Can you work these out from the model? Positions are in its coordinate system, mm. A direction names the side the tool comes from. Coordinates: 2 decimals unless noted, no trailing zeros. Order: outer loops, then holes, each group sorted by start corner. A loop starts at its lowest first (then second) coordinate and runs counter-clockwise, first axis right, second up. Notation, with made-up numbers: (45.25, -4) -> (62.25, -4) arc R28 cw to (62.25, 21) -> close; hole circle Ø5 at (89.25, 16.5). An arc over 180 degrees is marked (long way). Answer as a JSON object with one key per item and string values. Group by question number.
(1) For pin 1 (1.9 mm diameter, centred on y = -3.5, z = 120, fed in from -X), with a flat end and sliding along its axis, tell me the tip position at first contact or that it passes through.
(2) I want a section at B-B, the plane z = 112.5. List the corners of the cut face in (x, y) for me.
(3) I want a section at C-C, the plane x = 69.5. List the corners of the cut face in (y, z) for me, plus the area to 3 significant figures.
(4) Which directions (+Z, -Z, +X, -X, +Y, -Y) give clear straight access to the entire face, cutting with the end or side of a thin tool? Please do faces 1 (the flat face through (44, -6.35, 155)), 2 (the flat face through (6.35, -3, 91)).
(5) I want a section at A-A, the plane y = -4. List the corners of the cut face in (x, z) for me (3 decimals).
(6) I need wall thicknesses on line 1 (X direction, y = -3.25, z = 102.5); line 2 (Z direction, x = 77, y = -2); line 3 (Z direction, x = 71.5, y = -5.75). Which ranges of each line are inside material? Lowest first, please.
from build123d import *

# Parameters (mm, degrees)
F0_W     = 95.25
F0_H     = 279.4
F1_DEPTH = 6.35
F3_DEPTH = 25.4
F5_DEPTH = 6.35
F7_DEPTH = 6.35


with BuildPart() as f1:
    # F0 (on Front) → F1 (new body)
    with BuildSketch(Plane.XZ):
        with Locations((47.625, 139.7)):
            Rectangle(F0_W, F0_H)
        Polygon((47.625, 304.8), (0, 279.4), (95.25, 279.4), align=None)
    extrude(amount=F1_DEPTH)

    # F2 (on face) → F3 (cut)
    with BuildSketch(Plane.XZ.offset(6.35)):
        Polygon((0, 0), (6.35, 0), (6.35, 177.8), (0, 182.2827526427), align=None)
    extrude(amount=-F3_DEPTH, mode=Mode.SUBTRACT)

    # F4 (on face) → F5 (cut)
    with BuildSketch(Plane.XZ.offset(6.35)):
        Polygon((0, 182.2827526427), (6.35, 177.8), (6.35, 185.5728740667), (0, 190.0556267094), align=None)
    extrude(amount=-F5_DEPTH, mode=Mode.SUBTRACT)

    # F6 (on face) → F7 (join)
    with BuildSketch(Plane.XZ.offset(6.35)):
        Polygon((0, 190.0556267094), (0, 279.4), (-6.35, 276.0133333333), (-6.35, 194.5383793521), align=None)
    extrude(amount=-F7_DEPTH)


solid = f1.part
Computed values:
{
 "1": {"pin 1": "stops at x = 6.35"},
 "2": {"outline": "(6.35, -6.35) -> (95.25, -6.35) -> (95.25, 0) -> (6.35, 0) -> close"},
 "3": {"outline": "(-6.35, 0) -> (0, 0) -> (0, 293.13) -> (-6.35, 293.13) -> close", "area": "1,860 mm2"},
 "4": {"face 1": "+Z, -Z, +X, -X, -Y", "face 2": "-Z, -X, +Y, -Y"},
 "5": {"outline": "(-6.35, 194.538) -> (6.35, 185.573) -> (6.35, 0) -> (95.25, 0) -> (95.25, 279.4) -> (47.625, 304.8) -> (-6.35, 276.013) -> close"},
 "6": {"line 1": "x = 6.35 to 95.25", "line 2": "z = 0 to 289.13", "line 3": "z = 0 to 292.07"}
}
